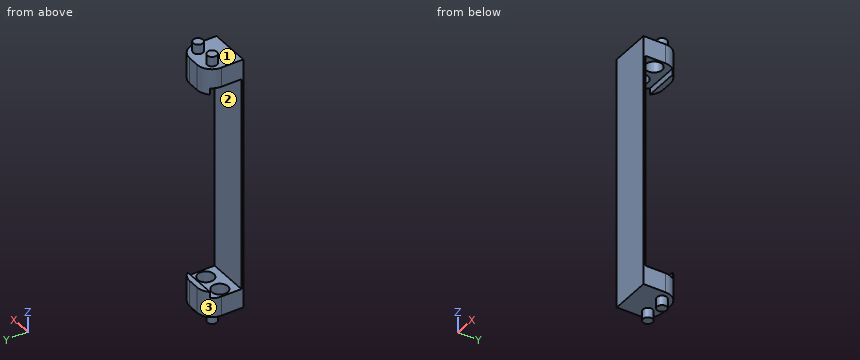
```python
from build123d import *

# Parameters (mm, degrees)
BOSS_EXTRUDE1_DEPTH      = 42
BOSS_EXTRUDE1_DEPTH_BACK = 42
FILLET1_R                = 30
CUT_EXTRUDE1_DEPTH       = 250
CUT_EXTRUDE1_DEPTH_BACK  = 250
SKETCH2_R                = 16.5
SKETCH3_R                = 10
BOSS_EXTRUDE2_DEPTH      = 20
BOSS_EXTRUDE3_START      = 20
SKETCH4_R                = 10
BOSS_EXTRUDE3_DEPTH      = 20


with BuildPart() as part:
    # Sketch1 → Boss-Extrude1 (new, two sides: drawn at the far end of the back side and taken through both)
    with BuildSketch(Plane(origin=(0, 0, 0), x_dir=(0, 0, -1), z_dir=(1, 0, 0)).offset(-BOSS_EXTRUDE1_DEPTH_BACK)):
        Polygon((-260, 0), (260, 0), (260, 75), (207, 75), (207, 64), (220, 64), (220, 4), (-220, 4), (-220, 64), (-207, 64), (-207, 75), (-260, 75), align=None)
    extrude(amount=BOSS_EXTRUDE1_DEPTH + BOSS_EXTRUDE1_DEPTH_BACK)

    # Fillet1
    fillet1_edges = [part.edges().sort_by_distance(p)[0] for p in [
        (-42, 75, -233.5),
        (42, 75, -233.5),
        (-42, 75, 233.5),
        (42, 75, 233.5),
    ]]
    fillet(fillet1_edges, radius=FILLET1_R)

    # Sketch2 → Cut-Extrude1 (cut, two sides: drawn at the far end of the back side and taken through both)
    with BuildSketch(Plane.XY.offset(-CUT_EXTRUDE1_DEPTH_BACK)):
        with Locations((22, 35)):
            Circle(SKETCH2_R)
        with Locations((-22, 35)):
            Circle(SKETCH2_R)
    extrude(amount=CUT_EXTRUDE1_DEPTH + CUT_EXTRUDE1_DEPTH_BACK, mode=Mode.SUBTRACT)

    # Sketch3 → Boss-Extrude2 (add)
    with BuildSketch(Plane.XY.offset(260)):
        with Locations((22, 51)):
            Circle(SKETCH3_R)
        with Locations((-22, 51)):
            Circle(SKETCH3_R)
    extrude(amount=BOSS_EXTRUDE2_DEPTH)

    # Sketch4 → Boss-Extrude3 (add)
    with BuildSketch(Plane(origin=(0, 0, -260), x_dir=(-1, 0, 0), z_dir=(0, 0, -1)).offset(BOSS_EXTRUDE3_START)):
        with Locations(Location((22, 51, 0), (0, 0, 180))):
            Circle(SKETCH4_R)
        with Locations(Location((-22, 51, 0), (0, 0, 180))):
            Circle(SKETCH4_R)
    extrude(amount=-BOSS_EXTRUDE3_DEPTH)


solid = part.part
```
Build history of the part. All positions in model axes, mm. Face numbers are marked on the shaded views. Coordinates: 2 decimals unless noted, no trailing zeros. Write each loop counter-clockwise with the first axis right and the second up, starting at its lowest first coordinate (ties: lowest second). Pieces come first, ordered by that corner, then holes.
1. Drop flat-ended pins along their axis: pin 1 (10 mm diameter, centred on x = 15, y = 32, fed in from +Z); pin 2 (10 mm diameter, centred on x = -29, z = -222.5, fed in from +Y); pin 3 (9 mm diameter, centred on x = -11, y = 68, fed in from -Z). Give the stop position or say it passes through.
Answer block:
pin 1: stops at z = 260
pin 2: stops at y = 72.5
pin 3: stops at z = -260
2. Pull direction Z, two halves, no side cores. Call the marked faces 1, 2 and 3: released by +Z, released by -Z, zero draft, split by the parting line, or undercut.
Answer block:
face 1: released by +Z
face 2: undercut
face 3: zero draft
3. Band-saw the part on D-D, the plane x = 17. Give the cut face in (y, z).
Answer block:
outline: (0, -260) - (42.34, -260) - (42.34, -280) - (59.66, -280) - (59.66, -260) - (74.58, -260) - (74.58, -207) - (64, -207) - (64, -220) - (50.72, -220) - (50.72, -250) - (19.28, -250) - (19.28, -220) - (4, -220) - (4, 220) - (19.28, 220) - (19.28, 250) - (50.72, 250) - (50.72, 220) - (64, 220) - (64, 207) - (74.58, 207) - (74.58, 260) - (59.66, 260) - (59.66, 280) - (42.34, 280) - (42.34, 260) - (0, 260) - close
4. Band-saw the part on B-B, the plane x = -22. Give the cut face in (y, z), and give its area (3 significant figures).
Answer block:
outline: (0, -260) - (41, -260) - (41, -280) - (61, -280) - (61, -260) - (73.28, -260) - (73.28, -207) - (64, -207) - (64, -220) - (51.5, -220) - (51.5, -250) - (18.5, -250) - (18.5, -220) - (4, -220) - (4, 220) - (18.5, 220) - (18.5, 250) - (51.5, 250) - (51.5, 220) - (64, 220) - (64, 207) - (73.28, 207) - (73.28, 260) - (61, 260) - (61, 280) - (41, 280) - (41, 260) - (0, 260) - close
area: 6,680 mm2
5. Band-saw the part on A-A, the plane y = 35. Give the cut face in (x, z).
Answer block:
outline: (-42, -260) - (42, -260) - (42, -220) - (38.5, -220) - (38.5, -250) - (5.5, -250) - (5.5, -220) - (-5.5, -220) - (-5.5, -250) - (-38.5, -250) - (-38.5, -220) - (-42, -220) - close; (-42, 220) - (-38.5, 220) - (-38.5, 250) - (-5.5, 250) - (-5.5, 220) - (5.5, 220) - (5.5, 250) - (38.5, 250) - (38.5, 220) - (42, 220) - (42, 260) - (-42, 260) - close
6. Band-saw the part on C-C, the plane z = 152.5. Give the cut face in (x, y), and give its area (3 significant figures).
Answer block:
outline: (-42, 0) - (42, 0) - (42, 4) - (-42, 4) - close
area: 336 mm2
7. Drill centre lines: probe 1 along X at (y, z) = (35, 231.25); probe 2 along Z at (x, y) = (13, 66); probe 3 along Z at (x, y) = (-9, 59). Where is each one in solid material? Low to high.
Answer block:
probe 1: x = -42 to -38.5, -5.5 to 5.5, 38.5 to 42
probe 2: z = -260 to -207, 207 to 260
probe 3: z = -260 to -220, 220 to 260
